Read the model definition and answer for the solid it produces. Units are mm, in the model's axes. Face numbers are marked on the shaded views. Round coordinates to 2 decimals unless told otherwise and drop trailing zeros. Write each loop counter-clockwise with the first axis right and the second up, starting at its lowest first coordinate (ties: lowest second). Pieces come first, ordered by that corner, then holes. Notation, with made-up numbers: (71.25, 26) -> (122.25, 26) arc R24 cw to (122.25, 49) -> close; hole circle Ø3 at (75, 42.5). An arc over 180 degrees is marked (long way). Return JSON: item names as keys, results as strings.
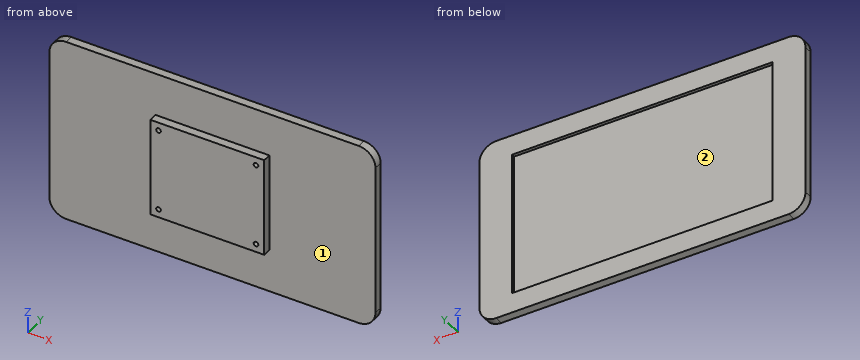
from build123d import *

# Parameters (mm, degrees)
SKETCH1_W           = 194
SKETCH1_H           = 110
BOSS_EXTRUDE1_DEPTH = 5
FILLET1_R           = 10
SKETCH2_W           = 155
SKETCH2_H           = 86
CUT_EXTRUDE1_DEPTH  = 2
SKETCH3_W           = 67.75
SKETCH3_H           = 58.75
SKETCH3_R           = 1.375
BOSS_EXTRUDE2_DEPTH = 5


with BuildPart() as part:
    # Sketch1 → Boss-Extrude1 (new body)
    with BuildSketch(Plane(origin=(0, 0, 0), x_dir=(1, 0, 0), z_dir=(0, 1, 0))):
        Rectangle(SKETCH1_W, SKETCH1_H)
    extrude(amount=-BOSS_EXTRUDE1_DEPTH)

    # Fillet1
    fillet1_edges = [part.edges().sort_by_distance(p)[0] for p in [
        (97, -2.5, 55),
        (-97, -2.5, 55),
        (-97, -2.5, -55),
        (97, -2.5, -55),
    ]]
    fillet(fillet1_edges, radius=FILLET1_R)

    # Sketch2 → Cut-Extrude1 (cut)
    with BuildSketch(Plane(origin=(0, 0, 0), x_dir=(1, 0, 0), z_dir=(0, 1, 0))):
        Rectangle(SKETCH2_W, SKETCH2_H)
    extrude(amount=-CUT_EXTRUDE1_DEPTH, mode=Mode.SUBTRACT)

    # Sketch3 → Boss-Extrude2 (add)
    with BuildSketch(Plane.XZ.offset(5)):
        Rectangle(SKETCH3_W, SKETCH3_H)
        with Locations(Location((-29, 24.5, 0), (0, 0, 270))):
            Circle(SKETCH3_R, mode=Mode.SUBTRACT)
        with Locations(Location((29, 24.5, 0), (0, 0, 270))):
            Circle(SKETCH3_R, mode=Mode.SUBTRACT)
        with Locations(Location((29, -24.5, 0), (0, 0, 270))):
            Circle(SKETCH3_R, mode=Mode.SUBTRACT)
        with Locations(Location((-29, -24.5, 0), (0, 0, 270))):
            Circle(SKETCH3_R, mode=Mode.SUBTRACT)
    extrude(amount=BOSS_EXTRUDE2_DEPTH)


solid = part.part
Item 1: Flat-ended cylindrical pins translate along their axes: pin 1 (10 mm diameter, centred on x = 46.5, z = -18.5, fed in from +Y); pin 2 (10 mm diameter, centred on x = -72.5, z = -33.5, fed in from -Y); pin 3 (4 mm diameter, centred on y = -8.5, z = 3, fed in from -X) (3 decimals); pin 4 (2 mm diameter, centred on x = -28.5, z = -24.5, fed in from -Y). Find the tip coordinate at first contact, or state that the pin passes through.
Worked answers:
{"pin 1": "stops at y = -2", "pin 2": "stops at y = -5", "pin 3": "stops at x = -33.875", "pin 4": "stops at y = -10"}
Item 2: Straight lines are drawn through the part: L1, parallel to X at y = -7.7, z = 24.5 (3 decimals); L2, parallel to Z at x = -5.5, y = -1; L3, parallel to Y at x = -50, z = 4. For each, find the intervals that lie inside material, in ascending order. Write a range as [from, to].
Worked answers:
{"L1": "x = [-33.875, -30.375], [-27.625, 27.625], [30.375, 33.875]", "L2": "z = [-55, -43], [43, 55]", "L3": "y = [-5, -2]"}
Item 3: Section B-B (x = -22) is taken. Give the vertices of the cut face in (y, z) (3 decimals).
Worked answers:
{"outline": "(-10, -29.375) -> (-5, -29.375) -> (-5, -55) -> (0, -55) -> (0, -43) -> (-2, -43) -> (-2, 43) -> (0, 43) -> (0, 55) -> (-5, 55) -> (-5, 29.375) -> (-10, 29.375) -> close"}
Item 4: For a pull along Z with two mould halves and no side action, classify the marked faces 1 and 2 as released by +Z, released by -Z, zero draft, split by the parting line, or undercut.
Worked answers:
{"face 1": "zero draft", "face 2": "undercut"}
Item 5: Section C-C (z = 39.5) is taken. Give the vertices of the cut face in (x, y).
Worked answers:
{"outline": "(-97, -5) -> (97, -5) -> (97, 0) -> (77.5, 0) -> (77.5, -2) -> (-77.5, -2) -> (-77.5, 0) -> (-97, 0) -> close"}
Item 6: Section A-A (z = 13.5) is taken. Give the vertices of the cut face in (x, y) (3 decimals).
Worked answers:
{"outline": "(-97, -5) -> (-33.875, -5) -> (-33.875, -10) -> (33.875, -10) -> (33.875, -5) -> (97, -5) -> (97, 0) -> (77.5, 0) -> (77.5, -2) -> (-77.5, -2) -> (-77.5, 0) -> (-97, 0) -> close"}
